```python
from build123d import *

# Parameters (mm, degrees)
F1_DEPTH = 3.175
F2_DEPTH = 9.525
F3_DEPTH = 9.525
F4_DEPTH = 6.35


with BuildPart() as f1:
    # F0 (on Top) → F1 (new body)
    with BuildSketch(Plane.XY):
        Polygon((0, 12.7), (0, 0), (7.62, 0), (7.62, -12.7), (15.24, -12.7), (15.24, 0), (21.59, 0), (21.59, -12.7), (29.21, -12.7), (29.21, 0), (35.56, 0), (35.56, -12.7), (43.18, -12.7), (43.18, 0), (50.8, 0), (50.8, 12.7), (33.655, 12.7), (33.655, 25.4), (26.035, 25.4), (26.035, 12.7), (18.415, 12.7), (18.415, 25.4), (10.795, 25.4), (10.795, 12.7), align=None)
    extrude(amount=F1_DEPTH)

    # F2 (cut): faces of the model
    f2_faces = [f1.faces().sort_by_distance(p)[0] for p in [
        (14.605, 25.4, 1.5875),
        (29.845, 25.4, 1.5875),
    ]]
    extrude(f2_faces, amount=-F2_DEPTH, mode=Mode.SUBTRACT)

    # F3 (cut): faces of the model
    f3_faces = [f1.faces().sort_by_distance(p)[0] for p in [
        (39.37, -12.7, 1.5875),
        (25.4, -12.7, 1.5875),
        (11.43, -12.7, 1.5875),
    ]]
    extrude(f3_faces, amount=-F3_DEPTH, mode=Mode.SUBTRACT)

    # F4 (add): faces of the model
    f4_faces = [f1.faces().sort_by_distance(p)[0] for p in [
        (42.2275, 12.7, 1.5875),
        (29.845, 15.875, 1.5875),
        (22.225, 12.7, 1.5875),
        (14.605, 15.875, 1.5875),
        (5.3975, 12.7, 1.5875),
    ]]
    extrude(f4_faces, amount=F4_DEPTH)


solid = f1.part
```
Build history of the part. All positions in model axes, mm. A direction names the side the tool comes from. Round coordinates to 2 decimals unless told otherwise and drop trailing zeros. Loops run counter-clockwise (first coordinate to the right, second up) from the corner with the lowest first, then second, coordinate; pieces in that order, holes last.
Item 1: Two-plate mould, pull along X, no slides. Class faces 1 (the face through (26, 9, 0)), 2 (the face through (21.59, -2, 2)), 3 (the face through (33.655, 21, 2)): released by +X, released by -X, zero draft, split by the parting line, or undercut.
Item 2: Saw through at C-C (z = 2.65). List the corners of the cut face in (x, y) (3 decimals), then the cut area to 3 significant figures.
Item 3: Drill centre lines: line 1 along X through (y, z) = (19.75, 2.15) (3 decimals); line 2 along Y through (x, z) = (4, 0.2); line 3 along Y through (x, z) = (30, 2.4) (3 decimals). Where is each one in solid material? Low to high.
Item 4: Saw through at D-D (x = 47). List the corners of the cut face in (y, z) (3 decimals).
Item 5: Pin check, flat tips, straight feed: P1, Ø1, axis at y = 20.5, z = 1.5, coming from the -X side (3 decimals); P2, Ø1, axis at y = -2, z = 1.5, coming from the -X side; P3, Ø1.6, axis at y = -1.5, z = 1, coming from the +X side. Stop position of each tip, or through.
Item 6: Saw through at A-A (y = -0.75). List the corners of the cut face in (x, z) (3 decimals).
Item 7: Saw through at B-B (y = 20.25). List the corners of the cut face in (x, z) (3 decimals).
Item 8: Which spindle directions (+Z, -Z, +X, -X, +Y, -Y) get a long thin tool onto all of the face, cutting with end or side? Do faces 4 (the face through (50.8, 9, 2)), 5 (the face through (26.035, 21, 2)), 6 (the face through (10.795, 21, 2)), 7 (the face through (4, 0, 2)), 8 (the face through (32, 0, 2)). Say none if no direction does.
Worked answers:
1. face 1: zero draft
1. face 2: undercut
1. face 3: released by +X
2. outline: (0, 0) - (7.62, 0) - (7.62, -3.175) - (15.24, -3.175) - (15.24, 0) - (21.59, 0) - (21.59, -3.175) - (29.21, -3.175) - (29.21, 0) - (35.56, 0) - (35.56, -3.175) - (43.18, -3.175) - (43.18, 0) - (50.8, 0) - (50.8, 19.05) - (33.655, 19.05) - (33.655, 22.225) - (26.035, 22.225) - (26.035, 19.05) - (18.415, 19.05) - (18.415, 22.225) - (10.795, 22.225) - (10.795, 19.05) - (0, 19.05) - close
2. area: 1,090 mm2
3. line 1: x = 10.795 to 18.415, 26.035 to 33.655
3. line 2: y = 0 to 19.05
3. line 3: y = 0 to 22.225
4. outline: (0, 0) - (19.05, 0) - (19.05, 3.175) - (0, 3.175) - close
5. P1: stops at x = 10.795
5. P2: stops at x = 7.62
5. P3: stops at x = 43.18
6. outline: (7.62, 0) - (15.24, 0) - (15.24, 3.175) - (7.62, 3.175) - close; (21.59, 0) - (29.21, 0) - (29.21, 3.175) - (21.59, 3.175) - close; (35.56, 0) - (43.18, 0) - (43.18, 3.175) - (35.56, 3.175) - close
7. outline: (10.795, 0) - (18.415, 0) - (18.415, 3.175) - (10.795, 3.175) - close; (26.035, 0) - (33.655, 0) - (33.655, 3.175) - (26.035, 3.175) - close
8. face 4: +Z, -Z, +X, +Y, -Y
8. face 5: +Z, -Z, +Y
8. face 6: +Z, -Z, -X, +Y
8. face 7: +Z, -Z, -X, -Y
8. face 8: +Z, -Z, -Y
